Verification items for the finished model (mm, model axes). A direction names the side the tool comes from. Give positions to 0.01 mm unless a question says otherwise; leave off trailing zeros. Loops run counter-clockwise (first coordinate to the right, second up) from the corner with the lowest first, then second, coordinate; pieces in that order, holes last. Notation, with made-up numbers: M -28,36 L -12,36 A23 ccw -12,49 Z; hole C -5,56 d1. An arc over 180 degrees is marked long. Use CSV: the item, a comma, the result in double quotes.
from build123d import *

# Parameters (mm, degrees)
BOSS_EXTRUDE1_DEPTH                  = 330.200001
BOSS_EXTRUDE1_DEPTH_BACK             = 330.200001
SKETCH3_W                            = 38.1
SKETCH3_H                            = 25.4
SKETCH3_W_2                          = 31.75
SKETCH3_H_2                          = 19.05
F_1_4_0_25_DIAMETER_HOLE2_AT_2_COUNT = 2
F_1_4_0_25_DIAMETER_HOLE2_AT_2_PITCH = 25.4
F_1_4_0_25_DIAMETER_HOLE2_AT_3_COUNT = 2
F_1_4_0_25_DIAMETER_HOLE2_AT_3_PITCH = 635.000000508
F_1_4_0_25_DIAMETER_HOLE2_AT_4_COUNT = 2
F_1_4_0_25_DIAMETER_HOLE2_AT_4_PITCH = 50.8
F_1_4_0_25_DIAMETER_HOLE2_AT_5_COUNT = 2
F_1_4_0_25_DIAMETER_HOLE2_AT_5_PITCH = 609.600000508
F_1_4_0_25_DIAMETER_HOLE3_D          = 6.35
F_13_64_0_20313_DIAMETER_HOLE1_D     = 5.159502
F_10_CLEARANCE_HOLE1_D               = 4.9784


with BuildPart() as part:
    # Sketch3 → Boss-Extrude1 (new, two sides: drawn at the far end of the back side and taken through both)
    with BuildSketch(Plane.XY.offset(-BOSS_EXTRUDE1_DEPTH_BACK)):
        Rectangle(SKETCH3_W, SKETCH3_H)
        Rectangle(SKETCH3_W_2, SKETCH3_H_2, mode=Mode.SUBTRACT)
    extrude(amount=BOSS_EXTRUDE1_DEPTH + BOSS_EXTRUDE1_DEPTH_BACK)

    # Sketch8 → 1/4 (0.25) Diameter Hole2 (revolve, cut)
    with BuildSketch(Plane(origin=(-19.05, 0, -317.500000508), x_dir=(0, 0, 1), z_dir=(0, 1, 0))):
        Polygon((0, 0), (0, 38.1), (3.9624, 38.1), (3.175, 37.194199916), (3.175, 0), align=None)
    f_1_4_0_25_diameter_hole2 = revolve(axis=Axis((-25.4, 0, -317.500000508), (1, 0, 0)), mode=Mode.SUBTRACT)

    # 1/4 (0.25) Diameter Hole2 at 2: 1/4 (0.25) Diameter Hole2 ×2
    with Locations(*[(0, 0, i * F_1_4_0_25_DIAMETER_HOLE2_AT_2_PITCH) for i in range(1, F_1_4_0_25_DIAMETER_HOLE2_AT_2_COUNT)]):
        add(f_1_4_0_25_diameter_hole2, mode=Mode.SUBTRACT)

    # 1/4 (0.25) Diameter Hole2 at 3: 1/4 (0.25) Diameter Hole2 ×2
    with Locations(*[(0, 0, i * F_1_4_0_25_DIAMETER_HOLE2_AT_3_PITCH) for i in range(1, F_1_4_0_25_DIAMETER_HOLE2_AT_3_COUNT)]):
        add(f_1_4_0_25_diameter_hole2, mode=Mode.SUBTRACT)

    # 1/4 (0.25) Diameter Hole2 at 4: 1/4 (0.25) Diameter Hole2 ×2
    with Locations(*[(0, 0, i * F_1_4_0_25_DIAMETER_HOLE2_AT_4_PITCH) for i in range(1, F_1_4_0_25_DIAMETER_HOLE2_AT_4_COUNT)]):
        add(f_1_4_0_25_diameter_hole2, mode=Mode.SUBTRACT)

    # 1/4 (0.25) Diameter Hole2 at 5: 1/4 (0.25) Diameter Hole2 ×2
    with Locations(*[(0, 0, i * F_1_4_0_25_DIAMETER_HOLE2_AT_5_PITCH) for i in range(1, F_1_4_0_25_DIAMETER_HOLE2_AT_5_COUNT)]):
        add(f_1_4_0_25_diameter_hole2, mode=Mode.SUBTRACT)

    # 1/4 (0.25) Diameter Hole3 (through all)
    with Locations(Plane(origin=(19.05, 0, 0), x_dir=(0, 0, -1), z_dir=(1, 0, 0))):
        with Locations((-266.7, 0), (-241.3, 0), (-215.9, 0), (241.300000508, 0), (215.900000508, 0), (190.500000508, 0)):
            Hole(F_1_4_0_25_DIAMETER_HOLE3_D / 2)

    # 13/64 (0.20313) Diameter Hole1 (through all)
    with Locations(Plane(origin=(19.05, 0, 0), x_dir=(0, 0, -1), z_dir=(1, 0, 0))):
        with Locations((152.4, 0), (-177.8, 0)):
            Hole(F_13_64_0_20313_DIAMETER_HOLE1_D / 2)

    # #10 Clearance Hole1 (through all)
    with Locations(Plane.ZY.offset(19.05)):
        with Locations((-120.650000508, 0), (146.05, 0)):
            Hole(F_10_CLEARANCE_HOLE1_D / 2)


solid = part.part
(1) Mould release check, pull along X, two halves, no side actions. Record for faces 1 (the flat face through (19.05, 0, -5)), 2 (the flat face through (15.875, 0, -5)), 3 (the flat face through (0, 12.7, -5)), 4 (the flat face through (0, 9.525, -5)): released by +X, released by -X, zero draft, split by the parting line, or undercut.
Calculated:
face 1,"released by +X"
face 2,"undercut"
face 3,"zero draft"
face 4,"undercut"
(2) Section check A-A on x = 1.5. Record the cut outline in (y, z) (3 decimals), plus the area to 3 significant figures.
Calculated:
outline,"M -12.7,-330.2 L -9.525,-330.2 L -9.525,330.2 L -12.7,330.2 Z; M 9.525,-330.2 L 12.7,-330.2 L 12.7,330.2 L 9.525,330.2 Z"
area,"4,190 mm²"
(3) Tool access check on faces 5 (the flat face through (-15.875, 0, -5)), 6 (the flat face through (0, -11, -330.2)). Record the directions out of +Z, -Z, +X, -X, +Y, -Y that give a thin tool (end or side, any length) a straight path to the whole face; none if there is none.
Calculated:
face 5,"+Z, -Z"
face 6,"-Z, +X, -X, +Y, -Y"
(4) Section check B-B on z = 279. Record the cut outline in (x, y) (3 decimals).
Calculated:
outline,"M -19.05,-12.7 L 19.05,-12.7 L 19.05,12.7 L -19.05,12.7 Z; hole M -15.875,-9.525 L 15.875,-9.525 L 15.875,9.525 L -15.875,9.525 Z"
(5) Scan lines: L1, parallel to X at y = 8, z = 235 (3 decimals); L2, parallel to Y at x = -17.35, z = -317.5 (3 decimals); L3, parallel to Y at x = -17, z = 146.05. Record each from-to range of solid material in increasing order. Write a range as from..to.
Calculated:
L1,"x = -19.05..-15.875, 15.875..19.05"
L2,"y = -12.7..-3.175, 3.175..12.7"
L3,"y = -12.7..-2.49, 2.49..12.7"
